Could you check a few things on this model? Use its own coordinates, in mm. A direction names the side the tool comes from. Give positions to 0.01 mm unless a question says otherwise; leave off trailing zeros. Write each loop counter-clockwise with the first axis right and the second up, starting at its lowest first coordinate (ties: lowest second). Pieces come first, ordered by that corner, then holes. Notation, with made-up numbers: M 65.25,80.5 L 73.25,80.5 A20 ccw 73.25,94.5 Z; hole C 4.25,52 d8. An arc over 180 degrees is marked long. One line per item, written item: value.
```python
from build123d import *

# Parameters (mm, degrees)
BASE_FLANGE1_DEPTH = 15.875
FILLET1_RADIUS     = 15.875
FILLET1_LENGTH     = 3.175
FILLET2_RADIUS     = 15.875
FILLET2_LENGTH     = 3.175
SKETCH6_R          = 3.175
CUT_EXTRUDE1_DEPTH = 48.625
SKETCH7_R          = 6.35
CUT_EXTRUDE2_DEPTH = 48.625
SKETCH8_R          = 2.0828
CUT_EXTRUDE3_DEPTH = 48.625


# Sheet-metal steps are written as plain solids
with BuildPart() as part:
    # Sketch1 → Base-Flange1 (new, symmetric)
    with BuildSketch(Plane.XY):
        with BuildLine():
            Line((0, 31.75), (0, 0.7366))
            ThreePointArc((0, 0.7366), (0.215745145, 0.215745145), (0.7366, 0))
            Line((0.7366, 0), (31.75, 0))
            Line((31.75, 0), (31.75, -3.175))
            Line((31.75, -3.175), (0.7366, -3.175))
            ThreePointArc((0.7366, -3.175), (-2.029318885, -2.029318885), (-3.175, 0.7366))
            Line((-3.175, 0.7366), (-3.175, 31.75))
            Line((-3.175, 31.75), (0, 31.75))
        make_face()
    extrude(amount=BASE_FLANGE1_DEPTH, both=True)

    # Fillet1: full round fillet: the end face becomes a half cylinder, R = half its width
    fillet1_face = Plane((-1.5875, 31.75, 0), x_dir=(1, 0, 0), z_dir=(0, 1, 0))  # on the end face: x along it, z out of the body
    fillet1_slab = fillet1_face.offset(-FILLET1_RADIUS / 2) * Box(FILLET1_LENGTH, 2 * FILLET1_RADIUS, FILLET1_RADIUS, mode=Mode.PRIVATE)  # the body's end, R deep
    fillet1_round = Plane((-1.5875, 15.875, 0), x_dir=(0, 1, 0), z_dir=(1, 0, 0)) * Cylinder(FILLET1_RADIUS, FILLET1_LENGTH, mode=Mode.PRIVATE)  # its axis R under the face
    add(fillet1_slab - fillet1_round, mode=Mode.SUBTRACT)

    # Fillet2: full round fillet: the end face becomes a half cylinder, R = half its width
    fillet2_face = Plane((31.75, -1.5875, 0), x_dir=(0, -1, 0), z_dir=(1, 0, 0))  # on the end face: x along it, z out of the body
    fillet2_slab = fillet2_face.offset(-FILLET2_RADIUS / 2) * Box(FILLET2_LENGTH, 2 * FILLET2_RADIUS, FILLET2_RADIUS, mode=Mode.PRIVATE)  # the body's end, R deep
    fillet2_round = Plane((15.875, -1.5875, 0), x_dir=(1, 0, 0), z_dir=(0, -1, 0)) * Cylinder(FILLET2_RADIUS, FILLET2_LENGTH, mode=Mode.PRIVATE)  # its axis R under the face
    add(fillet2_slab - fillet2_round, mode=Mode.SUBTRACT)

    # Sketch6 → Cut-Extrude1 (cut, through all)
    with BuildSketch(Plane(origin=(0, 0, 0), x_dir=(0, 0, -1), z_dir=(1, 0, 0))):
        with Locations(Location((0, 15.875, 0), (0, 0, 90))):
            Circle(SKETCH6_R)
    extrude(amount=-CUT_EXTRUDE1_DEPTH, mode=Mode.SUBTRACT)

    # Sketch7 → Cut-Extrude2 (cut, through all)
    with BuildSketch(Plane(origin=(0, 0, 0), x_dir=(1, 0, 0), z_dir=(0, 1, 0))):
        with Locations(Location((15.875, 0, 0), (0, 0, 270))):
            Circle(SKETCH7_R)
    extrude(amount=-CUT_EXTRUDE2_DEPTH, mode=Mode.SUBTRACT)

    # Sketch8 → Cut-Extrude3 (cut, through all)
    with BuildSketch(Plane(origin=(0, 0, 0), x_dir=(1, 0, 0), z_dir=(0, 1, 0))):
        with Locations(Location((22.86, -6.985, 0), (0, 0, 270))):
            Circle(SKETCH8_R)
        with Locations(Location((22.86, 6.985, 0), (0, 0, 270))):
            Circle(SKETCH8_R)
        with Locations(Location((8.89, 6.985, 0), (0, 0, 270))):
            Circle(SKETCH8_R)
        with Locations(Location((8.89, -6.985, 0), (0, 0, 270))):
            Circle(SKETCH8_R)
    extrude(amount=-CUT_EXTRUDE3_DEPTH, mode=Mode.SUBTRACT)


solid = part.part
```
1) On a 3-axis mill with a long thin cutter (end or side, diameter ignored), from which of +Z, -Z, +X, -X, +Y, -Y can I reach the whole of each face in a straight line? I mean faces 1 (the face through (-3.175, 16, 4)), 2 (the face through (9, 0, 0)). Say none if no direction works.
Outcome:
face 1: +Z, -Z, -X, +Y, -Y
face 2: +Z, -Z, +X, +Y
2) Please list where these lines run through material, in increasing order: L1, parallel to X at y = 26.5, z = -5 (3 decimals); L2, parallel to Z at x = -2, y = 14 (3 decimals). Write a range as from..to.
Outcome:
L1: x = -3.175..0
L2: z = -15.875..-2.562, 2.562..15.875
3) If we section it at A-A, the plane z = 0: Write out the boundary of the cut face in (x, y) (3 decimals).
Outcome:
outline: M -3.175,0.737 A3.912 ccw 0.737,-3.175 L 9.525,-3.175 L 9.525,0 L 0.737,0 A0.737 cw 0,0.737 L 0,12.7 L -3.175,12.7 Z; M -3.175,19.05 L 0,19.05 L 0,31.75 L -3.175,31.75 Z; M 22.225,-3.175 L 31.75,-3.175 L 31.75,0 L 22.225,0 Z
4) If we section it at B-B, the plane x = 8.89: Write out the boundary of the cut face in (y, z) (3 decimals), then the cut area to 3 significant figures.
Outcome:
outline: M -3.175,-15.875 L 0,-15.875 L 0,-9.068 L -3.175,-9.068 Z; M -3.175,-4.902 L 0,-4.902 L 0,4.902 L -3.175,4.902 Z; M -3.175,9.068 L 0,9.068 L 0,15.875 L -3.175,15.875 Z
area: 74.4 mm^2
5) We'd pull the mould along Z, two halves only. Please class faces 3 (the face through (4, -1, -15.875)), 4 (the face through (9.676, -1.565, -1.377)), 5 (the face through (-2, -2.06, 0.22)): pulls with the +Z half, pulls with the -Z half, needs draft (parallel to the pull), parting line crosses it, or undercut.
Outcome:
face 3: pulls with the -Z half
face 4: undercut
face 5: needs draft
6) I'm going to push flat-ended pins straight in: pin 1 (9.5 mm diameter, centred on x = 20, z = 7.5, fed in from +Y); pin 2 (5.5 mm diameter, centred on x = 22.86, z = 6.985, fed in from -Y) (3 decimals); pin 3 (7.5 mm diameter, centred on y = 15.875, z = 0, fed in from +X). Where does each tip first touch, or does it pass through?
Outcome:
pin 1: stops at y = 0
pin 2: stops at y = -3.175
pin 3: stops at x = 0
7) If we section it at D-D, the plane z = 11: Write out the boundary of the cut face in (x, y) (3 decimals).
Outcome:
outline: M -3.175,0.737 A3.912 ccw 0.737,-3.175 L 27.321,-3.175 L 27.321,0 L 0.737,0 A0.737 cw 0,0.737 L 0,27.321 L -3.175,27.321 Z
8) If we section it at C-C, the plane y = 14: Write out the boundary of the cut face in (x, z) (3 decimals).
Outcome:
outline: M -3.175,-15.875 L 0,-15.875 L 0,-2.562 L -3.175,-2.562 Z; M -3.175,2.562 L 0,2.562 L 0,15.875 L -3.175,15.875 Z
